from build123d import *

# Parameters (mm, degrees)
SKETCH_1_W          = 34
SKETCH_1_H          = 12
SKETCH_1_R          = 1.5
EXTRUDE_4_DEPTH     = 4
SKETCH_4_W          = 34
SKETCH_4_H          = 4
EXTRUDE_5_DEPTH     = 15
SKETCH_5_R          = 1.25
SKETCH_5_W          = 23.5
SKETCH_5_H          = 10
CUT_EXTRUDE_1_DEPTH = 40.761790704
FILLET_4_R          = 1
FILLET_6_R          = 2
FILLET_7_R          = 2
FILLET_8_R          = 1
FILLET_9_R          = 1
FILLET_10_R         = 1
FILLET_11_R         = 1


with BuildPart() as part:
    # 草图1 → 凸台-拉伸4 (new body)
    with BuildSketch(Plane(origin=(0, 0, 0), x_dir=(1, 0, 0), z_dir=(0, 1, 0))):
        with Locations((17, -6)):
            Rectangle(SKETCH_1_W, SKETCH_1_H)
        with Locations(Location((4.5, -8, 0), (0, 0, 270))):
            Circle(SKETCH_1_R, mode=Mode.SUBTRACT)
        with Locations(Location((29.5, -8, 0), (0, 0, 270))):
            Circle(SKETCH_1_R, mode=Mode.SUBTRACT)
    extrude(amount=EXTRUDE_4_DEPTH)

    # 草图4 → 凸台-拉伸5 (add)
    with BuildSketch(Plane(origin=(0, 4, 0), x_dir=(1, 0, 0), z_dir=(0, 1, 0))):
        with Locations((17, -2)):
            Rectangle(SKETCH_4_W, SKETCH_4_H)
    extrude(amount=EXTRUDE_5_DEPTH)

    # 草图5 → 切除-拉伸1 (cut, through all)
    with BuildSketch(Plane.XY.offset(4)):
        with Locations((3, 16)):
            Circle(SKETCH_5_R)
        with Locations((31, 16)):
            Circle(SKETCH_5_R)
        with Locations((17, 14)):
            Rectangle(SKETCH_5_W, SKETCH_5_H)
    extrude(amount=-CUT_EXTRUDE_1_DEPTH, mode=Mode.SUBTRACT)

    # 圆角4
    fillet_4_edges = [part.edges().sort_by_distance(p)[0] for p in [
        (17, 4, 12),
    ]]
    fillet(fillet_4_edges, radius=FILLET_4_R)

    # 圆角6
    fillet_6_edges = [part.edges().sort_by_distance(p)[0] for p in [
        (0, 19, 2),
    ]]
    fillet(fillet_6_edges, radius=FILLET_6_R)

    # 圆角7
    fillet_7_edges = [part.edges().sort_by_distance(p)[0] for p in [
        (34, 19, 2),
    ]]
    fillet(fillet_7_edges, radius=FILLET_7_R)

    # 圆角8
    fillet_8_edges = [part.edges().sort_by_distance(p)[0] for p in [
        (5.25, 9, 2),
    ]]
    fillet(fillet_8_edges, radius=FILLET_8_R)

    # 圆角9
    fillet_9_edges = [part.edges().sort_by_distance(p)[0] for p in [
        (28.75, 9, 2),
    ]]
    fillet(fillet_9_edges, radius=FILLET_9_R)

    # 圆角10
    fillet_10_edges = [part.edges().sort_by_distance(p)[0] for p in [
        (5.25, 19, 2),
        (28.75, 19, 2),
    ]]
    fillet(fillet_10_edges, radius=FILLET_10_R)

    # 圆角11
    fillet_11_edges = [part.edges().sort_by_distance(p)[0] for p in [
        (17, 4, 4),
    ]]
    fillet(fillet_11_edges, radius=FILLET_11_R)


solid = part.part
Read the model definition and answer for the solid it produces. Units are mm, in the model's axes. A direction names the side the tool comes from. Coordinates: 2 decimals unless noted, no trailing zeros. Loops run counter-clockwise (first coordinate to the right, second up) from the corner with the lowest first, then second, coordinate; pieces in that order, holes last. Notation, with made-up numbers: (87.5, 73) -> (121.5, 73) arc R6 cw to (121.5, 84) -> close; hole circle Ø1 at (-23.5, -9). An arc over 180 degrees is marked (long way). Answer in a Markdown table with one row per item.
Item 1: A cutting plane is placed at C-C on y = 11. Determine the outline of the cut face in (x, z).
Returned:
| item | result |
|---|---|
| outline | (0, 0) -> (5.25, 0) -> (5.25, 4) -> (0, 4) -> close; (28.75, 0) -> (34, 0) -> (34, 4) -> (28.75, 4) -> close |
Item 2: For faces 4 (the flat face through (16.8, 8.8, 4)), 5 (the flat face through (0, 6, 3)), 6 (the cylindrical face through (5.551, 9.285, 1.972)), determine the directions among +Z, -Z, +X, -X, +Y, -Y from which every point of the face is accessible in a straight line to the end or side of a thin tool.
Returned:
| item | result |
|---|---|
| face 4 | +Z, +X, -X, +Y |
| face 5 | +Z, -Z, -X, +Y, -Y |
| face 6 | +Z, -Z, +Y |
Item 3: A cutting plane is placed at D-D on z = 3.25. Determine the outline of the cut face in (x, y).
Returned:
| item | result |
|---|---|
| outline | (0, 0) -> (34, 0) -> (34, 17) arc R2 ccw to (32, 19) -> (29.75, 19) arc R1 ccw to (28.75, 18) -> (28.75, 10) arc R1 cw to (27.75, 9) -> (6.25, 9) arc R1 cw to (5.25, 10) -> (5.25, 18) arc R1 ccw to (4.25, 19) -> (2, 19) arc R2 ccw to (0, 17) -> close; hole circle Ø2.5 at (3, 16); hole circle Ø2.5 at (31, 16) |
Item 4: A cutting plane is placed at A-A on y = 16. Determine the outline of the cut face in (x, z).
Returned:
| item | result |
|---|---|
| outline | (0, 0) -> (1.75, 0) -> (1.75, 4) -> (0, 4) -> close; (4.25, 0) -> (5.25, 0) -> (5.25, 4) -> (4.25, 4) -> close; (28.75, 0) -> (29.75, 0) -> (29.75, 4) -> (28.75, 4) -> close; (32.25, 0) -> (34, 0) -> (34, 4) -> (32.25, 4) -> close |
Item 5: For a pull along Y with two mould halves and no side action, classify faces 1 (the cylindrical face through (3.672, 17.054, 2.028)), 2 (the cylindrical face through (4.57, 1.97, 6.5)), 3 (the cylindrical face through (28.449, 9.285, 1.972)) as released by +Y, released by -Y, zero draft, split by the parting line, or undercut.
Returned:
| item | result |
|---|---|
| face 1 | undercut |
| face 2 | zero draft |
| face 3 | released by +Y |
Item 6: Each of these flat-tipped pins is pushed along its axis until it touches: P1, Ø3, axis at x = 16, z = 2.5, coming from the +Y side; P2, Ø11, axis at x = 23.5, y = 12.5, coming from the +Z side; P3, Ø5, axis at x = 10, z = 8, coming from the +Y side. Where does it stop, or does it pass through?
Returned:
| item | result |
|---|---|
| P1 | stops at y = 9 |
| P2 | stops at z = 4 |
| P3 | stops at y = 4 |
Item 7: Straight lines are drawn through the part: line 1 along X through (y, z) = (1.1, 8); line 2 along X through (y, z) = (16.5, 1); line 3 along X through (y, z) = (16.25, 3.5). For each, find the intervals that lie inside material, in ascending order. Write a range as [from, to].
Returned:
| item | result |
|---|---|
| line 1 | x = [0, 3], [6, 28], [31, 34] |
| line 2 | x = [0, 1.85], [4.15, 5.25], [28.75, 29.85], [32.15, 34] |
| line 3 | x = [0, 1.78], [4.22, 5.25], [28.75, 29.78], [32.22, 34] |
Item 8: A cutting plane is placed at B-B on z = 8. Determine the outline of the cut face in (x, y).
Returned:
| item | result |
|---|---|
| outline | (0, 0) -> (3, 0) -> (3, 4) -> (0, 4) -> close; (6, 0) -> (28, 0) -> (28, 4) -> (6, 4) -> close; (31, 0) -> (34, 0) -> (34, 4) -> (31, 4) -> close |
